```python
from build123d import *

# Parameters (mm, degrees)
SKETCH4_W           = 6
SKETCH4_H           = 20
SKETCH4_R           = 1.5
BOSS_EXTRUDE1_DEPTH = 3
SKETCH6_W           = 3
SKETCH6_H           = 5
BOSS_EXTRUDE2_DEPTH = 12
SKETCH7_R           = 1.7
CUT_EXTRUDE1_DEPTH  = 20.137659209


with BuildPart() as part:
    # Sketch4 → Boss-Extrude1 (new body)
    with BuildSketch(Plane.XY):
        with Locations((0, -1)):
            Rectangle(SKETCH4_W, SKETCH4_H)
        Circle(SKETCH4_R, mode=Mode.SUBTRACT)
        with Locations((0, -8)):
            Circle(SKETCH4_R, mode=Mode.SUBTRACT)
    extrude(amount=BOSS_EXTRUDE1_DEPTH)

    # Sketch6 → Boss-Extrude2 (add)
    with BuildSketch(Plane.XY.offset(3)):
        with Locations((0, 6.5)):
            Rectangle(SKETCH6_W, SKETCH6_H)
    extrude(amount=BOSS_EXTRUDE2_DEPTH)

    # Sketch7 → Cut-Extrude1 (cut, through all)
    with BuildSketch(Plane(origin=(1.5, 0, 0), x_dir=(0, 0, -1), z_dir=(1, 0, 0))):
        with Locations(Location((-12, 6.5, 0), (0, 0, 90))):
            Circle(SKETCH7_R)
    extrude(amount=-CUT_EXTRUDE1_DEPTH, mode=Mode.SUBTRACT)


solid = part.part
```
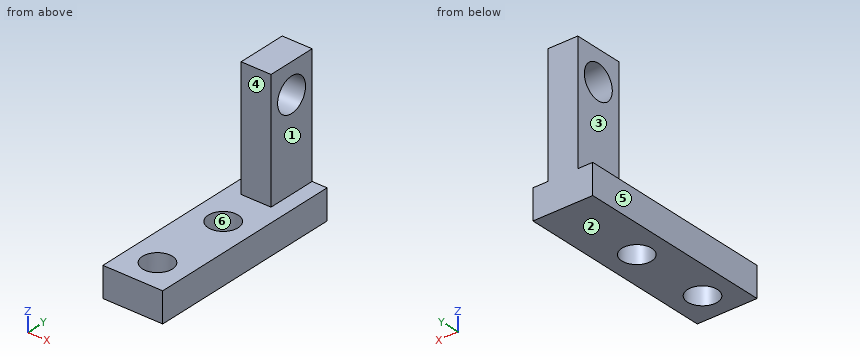
Build history of the part. All positions in model axes, mm. Face numbers are marked on the shaded views. A direction names the side the tool comes from. Round coordinates to 2 decimals unless told otherwise and drop trailing zeros. Write each loop counter-clockwise with the first axis right and the second up, starting at its lowest first coordinate (ties: lowest second). Pieces come first, ordered by that corner, then holes.
1) 3-axis set-ups, long thin cutter, end or side, ignore diameter. For the marked faces 1, 2 and 3: which of +Z, -Z, +X, -X, +Y, -Y reach the whole face in a straight line?
2) Mould opens along X. For the marked faces 4, 5 and 6 say: +X half, -X half, draft (parallel to the pull), parting line (faces both ways), or undercut.
3) Band-saw the part on B-B, the plane z = 12. List the corners of the cut face in (x, y).
4) Band-saw the part on D-D, the plane z = 1. List the corners of the cut face in (x, y), and give its area (3 significant figures).
5) Band-saw the part on C-C, the plane y = 0. List the corners of the cut face in (x, z), and give its area (3 significant figures).
6) Band-saw the part on A-A, the plane x = 0. List the corners of the cut face in (y, z), and give its area (3 significant figures).
7) Pin check, flat tips, straight feed: pin 1 (4 mm diameter, centred on y = 6.5, z = 12, fed in from +X); pin 2 (4 mm diameter, centred on y = 7.5, z = 10, fed in from -X); pin 3 (1.8 mm diameter, centred on x = 0, y = 0, fed in from -Z); pin 4 (1 mm diameter, centred on x = 0, y = -6.5, fed in from +Z). Stop position of each tip, or through.
8) Drill centre lines: probe 1 along Y at (x, z) = (0, 1.35); probe 2 along Z at (x, y) = (2.7, 5.25); probe 3 along Y at (x, z) = (0.5, 13.75). Where is each one in solid material? Low to high.
Ans:
1. face 1: +Z, +X, +Y, -Y
1. face 2: -Z, +X, -X, +Y, -Y
1. face 3: +Z, -X, +Y, -Y
2. face 4: draft
2. face 5: -X half
2. face 6: undercut
3. outline: (-1.5, 4) - (1.5, 4) - (1.5, 4.8) - (-1.5, 4.8) - close; (-1.5, 8.2) - (1.5, 8.2) - (1.5, 9) - (-1.5, 9) - close
4. outline: (-3, -11) - (3, -11) - (3, 9) - (-3, 9) - close; hole circle Ø3 at (0, -8); hole circle Ø3 at (0, 0)
4. area: 106 mm2
5. outline: (-3, 0) - (-1.5, 0) - (-1.5, 3) - (-3, 3) - close; (1.5, 0) - (3, 0) - (3, 3) - (1.5, 3) - close
5. area: 9.00 mm2
6. outline: (-11, 0) - (-9.5, 0) - (-9.5, 3) - (-11, 3) - close; (-6.5, 0) - (-1.5, 0) - (-1.5, 3) - (-6.5, 3) - close; (1.5, 0) - (9, 0) - (9, 15) - (4, 15) - (4, 3) - (1.5, 3) - close; hole circle Ø3.4 at (6.5, 12)
6. area: 92.9 mm2
7. pin 1: stops at x = 1.5
7. pin 2: stops at x = -1.5
7. pin 3: passes through
7. pin 4: stops at z = 3
8. probe 1: y = -11 to -9.5, -6.5 to -1.5, 1.5 to 9
8. probe 2: z = 0 to 3
8. probe 3: y = 4 to 9
